Autodesk Inventor part; units mm, degrees
ref_plane "YZ Plane" through (0, 0, 0) normal (1, 0, 0) x (0, 1, 0)
ref_plane "XZ Plane" through (0, 0, 0) normal (0, 1, 0) x (-1, 0, 0)
ref_plane "XY Plane" through (0, 0, 0) normal (0, 0, 1) x (1, 0, 0)
sketch "Sketch2" plane through (0, 0, 0) normal (0, 1, 0) x (-1, 0, 0)
  line L0 (-105, 105) -> (105, 105)
  line L1 (105, 105) -> (105, -105)
  line L2 (105, -105) -> (-105, -105)
  line L3 (-105, -105) -> (-105, 105)
  line L4 (-105, 105) -> (105, -105) construction
  line L5 (105, 105) -> (-105, -105) construction
  circle A0 centre (0, 0) radius 15.95
  dimension "d11" = 210
  dimension "d12" = 210
  dimension "d13" = 31.9
extrude "Extrusion2" add sketch "Sketch2" along normal blind 8
sketch "Sketch3" plane through (0, 0, 0) normal (0, -1, 0) x (1, 0, 0)
  point P0 (0, 0)
  point P1 (32, 0)
  dimension "d16" = 32
hole "Hole1" at (32, 0, 0) direction (0, 1, 0) diameter 4.5 depth 8 tip angle 118
pattern_circular "Circular Pattern1" count 4 over 360 about axis through (0, 0, 0) along (0, 1, 0) of "Hole1"
sketch "Sketch4" plane through (0, 0, 0) normal (0, -1, 0) x (1, 0, 0)
  circle A0 centre (0, 32) radius 2.25
  circle A1 centre (-32, 0) radius 2.25
  circle A2 centre (0, -32) radius 2.25
  circle A3 centre (32, 0) radius 2.25
  circle A4 centre (0, 0) radius 15.95
  line L0 (105, 105) -> (-105, 105)
  line L1 (-105, 105) -> (-105, -105)
  line L2 (-105, -105) -> (105, -105)
  line L3 (105, -105) -> (105, 105)
  line L4 (-105, -63) -> (-97, -63)
  line L5 (-97, -63) -> (-97, -21)
  line L6 (-97, -21) -> (-105, -21)
  line L7 (-105, -21) -> (-105, -63)
  line L8 (-105, 21) -> (-97, 21)
  line L9 (-97, 21) -> (-97, 63)
  line L10 (-97, 63) -> (-105, 63)
  line L11 (-105, 63) -> (-105, 21)
  line L12 (-97, -21) -> (-97, 21) construction
  line L13 (-97, 63) -> (-97, 105) construction
  line L14 (-97, -63) -> (-97, -105)
  dimension "d27" = 8
extrude "Extrusion3" cut sketch "Sketch4" against normal through all contours L10 L9 L8 L1 | L4 L1 L6 L5
sketch "Sketch5" plane through (0, 0, 0) normal (0, -1, 0) x (1, 0, 0)
  line L0 (-97, 21) -> (-105, 21)
  line L1 (-105, 21) -> (-105, -21)
  line L2 (-105, -21) -> (-97, -21)
  line L3 (-97, -21) -> (-97, -63)
  line L4 (-97, -63) -> (-105, -63)
  line L5 (-105, -63) -> (-105, -105)
  line L6 (-105, -105) -> (105, -105)
  line L7 (105, -105) -> (105, 105)
  line L8 (105, 105) -> (-105, 105)
  line L9 (-105, 105) -> (-105, 63)
  line L10 (-105, 63) -> (-97, 63)
  line L11 (-97, 63) -> (-97, 21)
  circle A0 centre (0, 32) radius 2.25
  circle A1 centre (-32, 0) radius 2.25
  circle A2 centre (0, -32) radius 2.25
  circle A3 centre (32, 0) radius 2.25
  circle A4 centre (0, 0) radius 15.95
  line L12 (63, -105) -> (21, -105)
  line L13 (21, -105) -> (21, -97)
  line L14 (21, -97) -> (63, -97)
  line L15 (63, -97) -> (63, -105)
  line L16 (-21, -105) -> (-63, -105)
  line L17 (-63, -105) -> (-63, -97)
  line L18 (-63, -97) -> (-21, -97)
  line L19 (-21, -97) -> (-21, -105)
  line L20 (63, -97) -> (105, -97) construction
  line L21 (21, -97) -> (-21, -97) construction
  line L22 (-63, -97) -> (-105, -97) construction
  dimension "d31" = 8
extrude "Extrusion4" cut sketch "Sketch5" against normal through all contours L6 L13 L14 L15 | L17 L18 L19 L6
mirror "Mirror1" about plane through (0, 0, 0) normal (1, 0, 0) of "Extrusion3"
mirror "Mirror2" about plane through (0, 0, 0) normal (0, 0, 1) of "Extrusion4"
equation "\"d11\" = d12"
properties part number "M01 - Base Top" material "Polycarbonate, Clear"
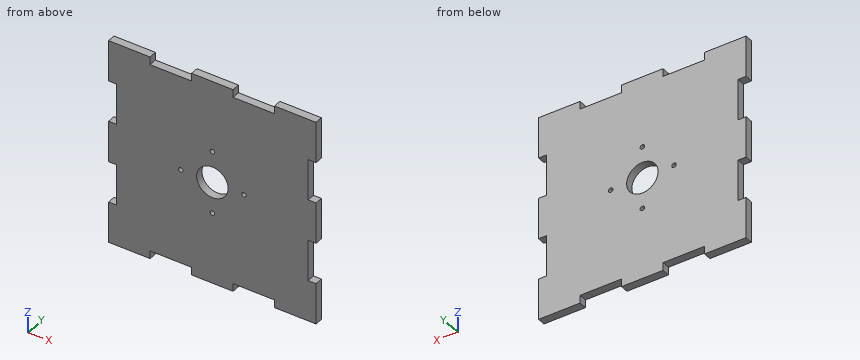
Source: CAD feature listing. Evaluate the final solid. Frame: model axes, mm. Round coordinates to 2 decimals unless told otherwise and drop trailing zeros. Write each loop counter-clockwise with the first axis right and the second up, starting at its lowest first coordinate (ties: lowest second). Pieces come first, ordered by that corner, then holes. Notation, with made-up numbers: M -23.75,-22.5 L 2.25,-22.5 A18 cw 2.25,0.5 Z; hole C -20,52 d11. An arc over 180 degrees is marked long. One line per item, written item: value. Start each with the question number.
Item 1: Section query A-A (y = 3.5). State how many separate pieces and enclosed holes the cut face has, plus the area to 3 significant figures.
Item 2: Pin query (flat end, axial travel): pin 1 (4 mm diameter, centred on y = 1.5, z = 59, fed in from +X); pin 2 (4 mm diameter, centred on x = 40, y = 2.5, fed in from -Z); pin 3 (2.5 mm diameter, centred on x = -32, z = 0, fed in from -Y); pin 4 (4 mm diameter, centred on y = 3.5, z = 42.5, fed in from -X). Return the tip coordinate at first contact, or that it passes through.
Item 3: Section query C-C (z = 24). Return the cut outline in (x, y).
Item 4: Ray query, L1, parallel to Z at x = 0, y = 5; L2, parallel to Z at x = 62.5, y = 1.25. Return the intervals inside material, ascending. Write a range as from..to.
Item 5: Section query B-B (x = -52). Return the cut outline in (y, z), plus the area to 3 significant figures.
Result set:
1. separate pieces: 1
1. enclosed holes: 5
1. area: 40,500 mm²
2. pin 1: stops at x = 97
2. pin 2: stops at z = -97
2. pin 3: passes through
2. pin 4: stops at x = -97
3. outline: M -97,0 L 97,0 L 97,8 L -97,8 Z
4. L1: z = -105..-34.25, -29.75..-15.95, 15.95..29.75, 34.25..105
4. L2: z = -97..97
5. outline: M 0,-97 L 8,-97 L 8,97 L 0,97 Z
5. area: 1,550 mm²
